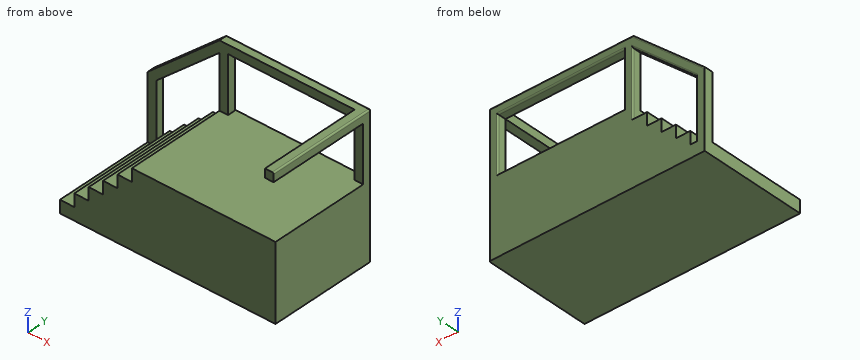
```python
from build123d import *

# Parameters (mm, degrees)
F1_DEPTH = 15
F2_DEPTH = 1.2
F3_W     = 1.2
F3_H     = 1.2
F4_DEPTH = 14.1
F5_R     = 0.2


# Not quite as in the source:
# - a feature names something its author has since deleted; it is built from what else it names


with BuildPart() as f1:
    # F0 (on Front) → F1 (new body)
    with BuildSketch(Plane.XZ):
        Polygon((-62.2959427714, 8.75), (-63.4959427714, 8.75), (-63.4959427714, 7), (-36.9959427714, 7), (-33.4959427714, 7), (-33.4959427714, 17.5), (-34.6959427714, 17.5), (-52.2959427714, 17.5), (-53.4959427714, 17.5), (-53.4959427714, 15.75), (-55.4959427714, 15.75), (-55.4959427714, 14), (-57.4959427714, 14), (-57.4959427714, 12.25), (-59.4959427714, 12.25), (-59.4959427714, 10.5), (-61.4959427714, 10.5), (-61.4959427714, 8.75), align=None)
    extrude(amount=F1_DEPTH)

    # F0 (on Front) → F2 (join)
    with BuildSketch(Plane.XZ):
        Polygon((-61.3689829591, 19.6110898358), (-63.4959427714, 17.75), (-63.4959427714, 17.0856158867), (-63.4959427714, 16.1554781281), (-62.2959427714, 17.2054781281), (-60.5787774297, 18.7079978021), align=None)
        Polygon((-62.2959427714, 17.2054781281), (-63.4959427714, 16.1554781281), (-63.4959427714, 8.75), (-62.2959427714, 8.75), align=None)
        Polygon((-52.2959427714, 26.5), (-53.4959427714, 26.5), (-53.4959427714, 24.9054781281), (-53.4959427714, 17.5), (-52.2959427714, 17.5), (-52.2959427714, 25.3), (-52.2959427714, 26), align=None)
        Polygon((-53.4959427714, 26.5), (-61.3689829591, 19.6110898358), (-60.5787774297, 18.7079978021), (-53.4959427714, 24.9054781281), align=None)
        Polygon((-34.6959427714, 26.5), (-52.2959427714, 26.5), (-52.2959427714, 26), (-52.2959427714, 25.3), (-34.6959427714, 25.3), align=None)
        Polygon((-33.4959427714, 26.5), (-34.6959427714, 26.5), (-34.6959427714, 25.3), (-34.6959427714, 17.5), (-33.4959427714, 17.5), align=None)
    extrude(amount=F2_DEPTH)

    # F3 (on face) → F4 (join)
    with BuildSketch(Plane.XZ.offset(1.2)):
        with Locations((-34.0959427714, 25.9)):
            Rectangle(F3_W, F3_H)
    extrude(amount=F4_DEPTH)

    # F5
    f5_edges = [f1.edges().sort_by_distance(p)[0] for p in [
        (-43.495943, 0, 25.3),
        (-34.695943, 0, 21.4),
        (-52.295943, 0, 21.4),
        (-57.895943, 0, 21.055478),
        (-53.495943, 0, 20.327739),
        (-62.295943, 0, 12.977739),
        (-58.495943, 0, 22.125),
        (-43.495943, 0, 26.5),
        (-33.495943, 0, 16.75),
        (-33.495943, -7.65, 26.5),
    ]]
    fillet(f5_edges, radius=F5_R)


solid = f1.part
```
Read the model definition and answer for the solid it produces. Units are mm, in the model's axes. Give positions to 0.01 mm unless a question says otherwise; leave off trailing zeros. Loops run counter-clockwise (first coordinate to the right, second up) from the corner with the lowest first, then second, coordinate; pieces in that order, holes last.
Item 1: Each of these flat-tipped pins is pushed along its axis until it touches: pin 1 Ø5.5 at (x, z) = (-51.5, 20.5) entering from -Y; pin 2 Ø0.5 at (y, z) = (-0.5, 21.5) entering from -X; pin 3 Ø1.4 at (y, z) = (-9, 13) entering from -X; pin 4 Ø4 at (y, z) = (-5.5, 18) entering from +X. Where does it stop, or does it pass through?
Item 2: The part is cut by section B-B (y = -14). Write down the section's boundary in (x, z).
Item 3: The part is cut by section A-A (z = 10). Write down the section's boundary in (x, y), and give its area (3 significant figures).
Item 4: The part is cut by section C-C (x = -37). Write down the section's boundary in (y, z), and give its area (3 significant figures).
Item 5: The part is cut by section D-D (y = -0.75). Write down the section's boundary in (x, z).
Item 6: Find the intervals of material crossed by line 1 along X through (y, z) = (-1, 17); line 2 along Z through (x, y) = (-62, -12.5); line 3 along Z through (x, y) = (-42, -0.75), in increasing order.
Taken from the geometry:
1. pin 1: stops at y = -1.2
1. pin 2: stops at x = -59.5
1. pin 3: stops at x = -57.5
1. pin 4: stops at x = -33.5
2. outline: (-63.5, 7) - (-33.5, 7) - (-33.5, 17.5) - (-53.5, 17.5) - (-53.5, 15.75) - (-55.5, 15.75) - (-55.5, 14) - (-57.5, 14) - (-57.5, 12.25) - (-59.5, 12.25) - (-59.5, 10.5) - (-61.5, 10.5) - (-61.5, 8.75) - (-63.5, 8.75) - close; (-34.7, 25.3) - (-33.5, 25.3) - (-33.5, 26.3) arc R0.2 ccw to (-33.7, 26.5) - (-34.7, 26.5) - close
3. outline: (-63.5, -1.2) - (-62.3, -1.2) - (-62.3, -0.2) arc R0.2 ccw to (-62.5, 0) - (-63.5, 0) - close; (-61.5, -15) - (-33.5, -15) - (-33.5, -0.2) arc R0.2 ccw to (-33.7, 0) - (-61.5, 0) - close
3. area: 421 mm2
4. outline: (-15, 7) - (0, 7) - (0, 17.5) - (-15, 17.5) - close; (-1.2, 25.3) - (-0.2, 25.3) arc R0.2 ccw to (0, 25.5) - (0, 26.3) arc R0.2 ccw to (-0.2, 26.5) - (-1.2, 26.5) - close
4. area: 159 mm2
5. outline: (-63.5, 7) - (-33.5, 7) - (-33.5, 26.3) arc R0.2 ccw to (-33.7, 26.5) - (-53.5, 26.5) - (-63.5, 17.75) - close; hole (-62.3, 8.75) - (-61.5, 8.75) - (-61.5, 10.5) - (-59.5, 10.5) - (-59.5, 12.25) - (-57.5, 12.25) - (-57.5, 14) - (-55.5, 14) - (-55.5, 15.75) - (-53.5, 15.75) - (-53.5, 24.91) - (-62.3, 17.21) - close; hole (-52.3, 17.5) - (-34.7, 17.5) - (-34.7, 25.3) - (-52.3, 25.3) - close
6. line 1: x = -63.5 to -62.3, -53.5 to -33.5
6. line 2: z = 7 to 8.75
6. line 3: z = 7 to 17.5, 25.3 to 26.5
